```python
from build123d import *

# Parameters (mm, degrees)
SKETCH1_W               = 80
SKETCH1_H               = 100
BOSS_EXTRUDE1_DEPTH     = 10
SKETCH2_R               = 6.25
BOSS_EXTRUDE2_DEPTH     = 15
CUT_EXTRUDE1_DEPTH      = 99.615414617
CUT_EXTRUDE1_DEPTH_BACK = 99.615414617
SKETCH3_W               = 15
SKETCH3_H               = 55


with BuildPart() as part:
    # Sketch1 → Boss-Extrude1 (new body)
    with BuildSketch(Plane(origin=(0, 0, 0), x_dir=(1, 0, 0), z_dir=(0, 1, 0))):
        Rectangle(SKETCH1_W, SKETCH1_H)
    extrude(amount=BOSS_EXTRUDE1_DEPTH)

    # Sketch2 → Boss-Extrude2 (add, symmetric)
    with BuildSketch(Plane(origin=(0, 0, 0), x_dir=(0, 0, -1), z_dir=(1, 0, 0))):
        with BuildLine():
            Line((-35, 10), (-19.091339118, 60.959930425))
            ThreePointArc((-19.091339118, 60.959930425), (0, 75), (19.091339118, 60.959930425))
            Line((19.091339118, 60.959930425), (35, 10))
            Line((35, 10), (-35, 10))
        make_face()
        with Locations((0, 55)):
            Circle(SKETCH2_R, mode=Mode.SUBTRACT)
    extrude(amount=BOSS_EXTRUDE2_DEPTH, both=True)

    # Sketch3 → Cut-Extrude1 (cut, two sides: drawn at the far end of the back side and taken through both)
    with BuildSketch(Plane.XY.offset(-CUT_EXTRUDE1_DEPTH_BACK)):
        with Locations((0, 47.5)):
            Rectangle(SKETCH3_W, SKETCH3_H)
    extrude(amount=CUT_EXTRUDE1_DEPTH + CUT_EXTRUDE1_DEPTH_BACK, mode=Mode.SUBTRACT)


solid = part.part
```
Geometry: final body of the model. Coordinates: model frame, mm. A direction names the side the tool comes from. Round coordinates to 2 decimals unless told otherwise and drop trailing zeros. Write each loop counter-clockwise with the first axis right and the second up, starting at its lowest first coordinate (ties: lowest second). Pieces come first, ordered by that corner, then holes.
Item 1: Section query D-D (y = 65). Return loops of the section in (x, z), plus the area to 3 significant figures.
Item 2: Section query A-A (z = 0). Return loops of the section in (x, y).
Item 3: Mould query, pull axis X, two halves, no side actions, for faces 1 (the face through (11, 75, 0)), 2 (the face through (7.5, 41, 0)), 3 (the face through (-15, 36, 0)), 4 (the face through (0, 20, 0)). Classes: +X half, -X half, draft (parallel to the pull), parting line (faces both ways), or undercut.
Item 4: Section query C-C (x = -1). Return loops of the section in (y, z).
Item 5: Pin query (flat end, axial travel): P1, Ø4, axis at x = -7.5, y = 28, coming from the -Z side; P2, Ø16.5, axis at y = 59, z = 10, coming from the +X side; P3, Ø12, axis at x = 16.5, y = 47, coming from the +Z side. Return the tip coordinate at first contact, or that it passes through.
Item 6: Material intervals for L1, parallel to X at y = 31, z = -24.5; L2, parallel to Y at x = 12.75, z = 0; L3, parallel to Y at x = -23, z = -19, sorted ascending.
Item 7: Set-up query: faces 5 (the face through (15, 36, 0)), 6 (the face through (-11, 75, 0)), 7 (the face through (-7.5, 41, 0)). Return all of +Z, -Z, +X, -X, +Y, -Y with unobstructed straight access to the full face (end or side cutting, diameter ignored); none if empty.
Item 8: Section query B-B (y = 55). Return loops of the section in (x, z), plus the area to 3 significant figures.
Completed:
1. outline: (-15, -17.32) - (-7.5, -17.32) - (-7.5, 17.32) - (-15, 17.32) - close; (7.5, -17.32) - (15, -17.32) - (15, 17.32) - (7.5, 17.32) - close
1. area: 520 mm2
2. outline: (-40, 0) - (40, 0) - (40, 10) - (15, 10) - (15, 48.75) - (7.5, 48.75) - (7.5, 20) - (-7.5, 20) - (-7.5, 48.75) - (-15, 48.75) - (-15, 10) - (-40, 10) - close; (-15, 61.25) - (-7.5, 61.25) - (-7.5, 75) - (-15, 75) - close; (7.5, 61.25) - (15, 61.25) - (15, 75) - (7.5, 75) - close
3. face 1: draft
3. face 2: undercut
3. face 3: -X half
3. face 4: undercut
4. outline: (0, -50) - (10, -50) - (10, -35) - (20, -31.88) - (20, 31.88) - (10, 35) - (10, 50) - (0, 50) - close
5. P1: stops at z = -30.01
5. P2: stops at x = 15
5. P3: stops at z = 25.26
6. L1: x = -15 to -7.5, 7.5 to 15
6. L2: y = 0 to 48.75, 61.25 to 75
6. L3: y = 0 to 10
7. face 5: +Z, -Z, +X, +Y
7. face 6: +X, -X, +Y
7. face 7: +Z, -Z, +Y
8. outline: (-15, -20.95) - (-7.5, -20.95) - (-7.5, -6.25) - (-15, -6.25) - close; (-15, 6.25) - (-7.5, 6.25) - (-7.5, 20.95) - (-15, 20.95) - close; (7.5, -20.95) - (15, -20.95) - (15, -6.25) - (7.5, -6.25) - close; (7.5, 6.25) - (15, 6.25) - (15, 20.95) - (7.5, 20.95) - close
8. area: 441 mm2
